Input: part model. Units: mm. Frame: model coordinates. A direction names the side the tool comes from. Round coordinates to 2 decimals unless told otherwise and drop trailing zeros. Order: outer loops, then holes, each group sorted by start corner. A loop starts at its lowest first (then second) coordinate and runs counter-clockwise, first axis right, second up.
Item 1: Cut plane D-D on z = 31. Output: boundary loops of the cut face in (x, y), then the cut area to 3 significant figures.
Item 2: Reachability of faces 1 (the cylindrical face through (109.723, 45.201, 49.115)), 2 (the cylindrical face through (85, 5, 55)), 3 (the flat face through (-44, 10, 55)) from +Z, -Z, +X, -X, +Y, -Y: full face, straight path, thin tool, end or side. Return the list, or none.
Item 3: Cut plane C-C on y = 28.5. Output: boundary loops of the cut face in (x, z), then the cut area to 3 significant figures.
Item 4: Cut plane B-B on x = 130. Output: boundary loops of the cut face in (y, z).
Item 5: Cut plane A-A on z = 16. Output: boundary loops of the cut face in (x, y).
Item 6: Mould query, pull axis Z, two halves, no side actions, for faces 4 (the flat face through (66, 5, 90)), 5 (the flat face through (-60, 5, 65)), 6 (the flat face through (66, 5, 20)). Classes: released by +Z, released by -Z, zero draft, split by the parting line, or undercut.
Item 7: First-contact query: pin 1 (11 mm diameter, centred on x = -35, y = 4.5, fed in from -Z); pin 2 (3 mm diameter, centred on x = 10.5, y = 25, fed in from +Z); pin 3 (4 mm diameter, centred on x = 73, z = 64, fed in from +Y). Flat tips, straight axial feed; report the tip coordinate or a pass-through.
Item 8: Line query: L1, parallel to X at y = 53, z = 55.5; L2, parallel to Z at x = 130, y = 22.5; L3, parallel to Z at x = 130, y = 49. Output: solid intervals per line, ascending.
```python
from build123d import *

# Parameters (mm, degrees)
BOSS_EXTRUDE1_DEPTH      = 110
CUT_EXTRUDE3_START       = -11
SKETCH3_W                = 42.087121525
SKETCH3_H                = 20
CUT_EXTRUDE3_DEPTH       = 27
BOSS_EXTRUDE4_DEPTH      = 20
BOSS_EXTRUDE4_DEPTH_BACK = 91
BOSS_EXTRUDE5_REACH      = 67
SKETCH8_R                = 21.258333205
SKETCH8_R_2              = 13.198570557
SKETCH9_R                = 13.198570557
CUT_EXTRUDE4_DEPTH       = 49


with BuildPart() as part:
    # Sketch2 → Boss-Extrude1 (new body)
    with BuildSketch(Plane.XY):
        with BuildLine():
            Line((-65, 0), (-19, 0))
            ThreePointArc((-19, 0), (0, 19), (19, 0))
            Line((19, 0), (65, 0))
            Line((65, 0), (65, 10))
            Line((65, 10), (22.912878475, 10))
            ThreePointArc((22.912878475, 10), (0, 25), (-22.912878475, 10))
            Line((-22.912878475, 10), (-65, 10))
            Line((-65, 10), (-65, 0))
        make_face()
    extrude(amount=BOSS_EXTRUDE1_DEPTH)

    # Sketch3 → Cut-Extrude3 (cut)
    with BuildSketch(Plane(origin=(0, 10, 0), x_dir=(1, 0, 0), z_dir=(0, 1, 0)).offset(CUT_EXTRUDE3_START)):
        with Locations((43.956439237, -10)):
            Rectangle(SKETCH3_W, SKETCH3_H)
        with BuildLine():
            Line((65, -55), (65, -45))
            Line((65, -45), (55, -45))
            ThreePointArc((55, -45), (45, -55), (55, -65))
            Line((55, -65), (65, -65))
            Line((65, -65), (65, -55))
        make_face()
        with Locations((43.956439237, -100)):
            Rectangle(SKETCH3_W, SKETCH3_H)
    cut_extrude3 = extrude(amount=CUT_EXTRUDE3_DEPTH, mode=Mode.SUBTRACT)

    # Mirror1: Cut-Extrude3 across plane
    add(cut_extrude3.mirror(Plane(origin=(0, 0, 0), x_dir=(0, 0, 1), z_dir=(1, 0, 0))), mode=Mode.SUBTRACT)

    # Sketch7 → Boss-Extrude4 (add, two sides)
    with BuildSketch(Plane(origin=(0, 0, 20), x_dir=(-1, 0, 0), z_dir=(0, 0, -1))) as boss_extrude4_sk:
        with BuildLine():
            Line((-25, 0), (-19, 0))
            ThreePointArc((-19, 0), (0, 19), (19, 0))
            Line((19, 0), (25, 0))
            ThreePointArc((25, 0), (0, 25), (-25, 0))
        make_face()
    extrude(amount=BOSS_EXTRUDE4_DEPTH)
    extrude(boss_extrude4_sk.sketch, amount=-BOSS_EXTRUDE4_DEPTH_BACK)

    # Sketch8 → Boss-Extrude5 (add, up to next)
    with BuildSketch(Plane(origin=(0, 65, 0), x_dir=(1, 0, 0), z_dir=(0, 1, 0)), mode=Mode.PRIVATE) as boss_extrude5_sk1:
        with Locations((0, -55.5)):
            Circle(SKETCH8_R)
        with Locations((0, -55.5)):
            Circle(SKETCH8_R_2, mode=Mode.SUBTRACT)
    boss_extrude5_tool1 = extrude(boss_extrude5_sk1.sketch, amount=-BOSS_EXTRUDE5_REACH, mode=Mode.PRIVATE) - part.part
    add(boss_extrude5_tool1.solids().sort_by_distance((-20.657057, 65, 55.5))[0])

    # Sketch9 → Cut-Extrude4 (cut)
    with BuildSketch(Plane(origin=(0, 65, 0), x_dir=(1, 0, 0), z_dir=(0, 1, 0))):
        with Locations((0, -55.5)):
            Circle(SKETCH9_R)
    extrude(amount=-CUT_EXTRUDE4_DEPTH, mode=Mode.SUBTRACT)

    # Mirror2: part across plane


with BuildPart() as part_1:
    add(part.part)
    add(part.part.mirror(Plane(origin=(65, 0, 0), x_dir=(0, 0, 1), z_dir=(1, 0, 0))))


solid = part_1.part
```
From the geometry:
1. outline: (-65, 0) - (-19, 0) arc R19 cw to (19, 0) - (111, 0) arc R19 cw to (149, 0) - (195, 0) - (195, 10) - (152.91, 10) arc R25 ccw to (107.09, 10) - (22.91, 10) arc R25 ccw to (-22.91, 10) - (-65, 10) - close
1. area: 2,460 mm2
2. face 1: +Y
2. face 2: +Y, -Y
2. face 3: +Z, -Z, -X, +Y
3. outline: circle Ø42.52 at (0, 55.5); circle Ø42.52 at (130, 55.5); hole circle Ø26.4 at (0, 55.5); hole circle Ø26.4 at (130, 55.5)
3. area: 1,740 mm2
4. outline: (19, 0) - (25, 0) - (25, 34.24) - (65, 34.24) - (65, 42.3) - (19, 42.3) - close; (19, 68.7) - (65, 68.7) - (65, 76.76) - (25, 76.76) - (25, 111) - (19, 111) - close
5. outline: (-25, 0) - (-19, 0) arc R19 cw to (19, 0) - (25, 0) arc R25 ccw to start; (105, 0) - (111, 0) arc R19 cw to (149, 0) - (155, 0) arc R25 ccw to start
6. face 4: released by +Z
6. face 5: undercut
6. face 6: released by -Z
7. pin 1: stops at z = 20
7. pin 2: stops at z = 74.76
7. pin 3: stops at y = 10
8. L1: x = -21.26 to -13.2, 13.2 to 21.26, 108.74 to 116.8, 143.2 to 151.26
8. L2: z = 0 to 42.3, 68.7 to 111
8. L3: z = 34.24 to 42.3, 68.7 to 76.76
